```python
from build123d import *

# Parameters (mm, degrees)
F0_W     = 2
F0_H     = 15
F0_W_2   = 20
F0_H_2   = 5
F1_DEPTH = 7.5
F2_START = 2.5
F0_H_3   = 20
F0_R     = 2.5
F0_H_4   = 4.9999991059
F2_DEPTH = 5
F3_START = -2.5
F3_DEPTH = 5


with BuildPart() as f1:
    # F0 (on Front) → F1 (new body, symmetric)
    with BuildSketch(Plane.XZ):
        Polygon((10, -10), (10, 35), (-10, 35), (-10, 17), (-10, 15), (-10, -10), align=None)
        with Locations((-3, 2.5)):
            Rectangle(F0_W, F0_H, mode=Mode.SUBTRACT)
        with Locations((-3, 22.5)):
            Rectangle(F0_W, F0_H, mode=Mode.SUBTRACT)
        with Locations((3, 2.5)):
            Rectangle(F0_W, F0_H, mode=Mode.SUBTRACT)
        with Locations((3, 22.5)):
            Rectangle(F0_W, F0_H, mode=Mode.SUBTRACT)
        with Locations((0, -12.5)):
            Rectangle(F0_W_2, F0_H_2)
    extrude(amount=F1_DEPTH, both=True)

    # F0 (on Front) → F2 (join)
    with BuildSketch(Plane.XZ.offset(F2_START)):
        with Locations((0, -12.5)):
            Rectangle(F0_W_2, F0_H_2)
        with Locations((0, -25)):
            Rectangle(F0_W_2, F0_H_3)
        with Locations((-5, -25)):
            Circle(F0_R, mode=Mode.SUBTRACT)
        with Locations((5, -25)):
            Circle(F0_R, mode=Mode.SUBTRACT)
        with Locations((0, -37.499999553)):
            Rectangle(F0_W_2, F0_H_4)
    extrude(amount=F2_DEPTH)

    # F0 (on Front) → F3 (join)
    with BuildSketch(Plane.XZ.offset(F3_START)):
        with Locations((0, -12.5)):
            Rectangle(F0_W_2, F0_H_2)
        with Locations((0, -25)):
            Rectangle(F0_W_2, F0_H_3)
        with Locations((-5, -25)):
            Circle(F0_R, mode=Mode.SUBTRACT)
        with Locations((5, -25)):
            Circle(F0_R, mode=Mode.SUBTRACT)
        with Locations((0, -37.499999553)):
            Rectangle(F0_W_2, F0_H_4)
    extrude(amount=-F3_DEPTH)


solid = f1.part
```
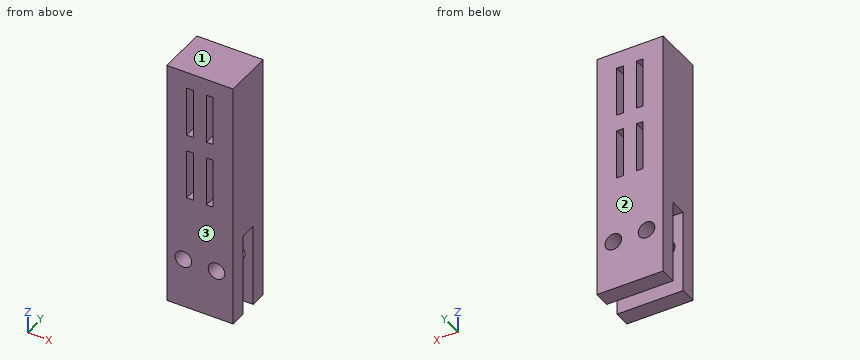
Source: CAD feature listing. Evaluate the final solid. Frame: model axes, mm. Face numbers are marked on the shaded views. Round coordinates to 2 decimals unless told otherwise and drop trailing zeros. Loops run counter-clockwise (first coordinate to the right, second up) from the corner with the lowest first, then second, coordinate; pieces in that order, holes last.
1. Section query D-D on y = -1.25. Output: boundary loops of the cut face in (x, z).
2. Section query C-C on z = -33. Output: boundary loops of the cut face in (x, y).
3. Mould query, pull axis Y, two halves, no side actions, for the marked faces 1, 2 and 3. Classes: released by +Y, released by -Y, zero draft, split by the parting line, or undercut.
4. Contact query for a flat-ended pin moving along its axis: pin 1 (2.5 mm diameter, centred on x = -2.5, y = 1, fed in from -Z). Output: stop coordinate, or through.
5. Ray query, L1, parallel to X at y = 3.75, z = 8; L2, parallel to Z at x = -2.25, y = -5.25; L3, parallel to Z at x = 2.25, y = -1.75. Return the intervals inside material, ascending.
6. Section query B-B on x = 5. Output: boundary loops of the cut face in (y, z).
7. Section query A-A on z = -25. Output: boundary loops of the cut face in (x, y), and give its area (3 significant figures).
Answers below:
1. outline: (-10, -15) - (10, -15) - (10, 35) - (-10, 35) - close; hole (-4, -5) - (-2, -5) - (-2, 10) - (-4, 10) - close; hole (-4, 15) - (-2, 15) - (-2, 30) - (-4, 30) - close; hole (2, -5) - (4, -5) - (4, 10) - (2, 10) - close; hole (2, 15) - (4, 15) - (4, 30) - (2, 30) - close
2. outline: (-10, -7.5) - (10, -7.5) - (10, -2.5) - (-10, -2.5) - close; (-10, 2.5) - (10, 2.5) - (10, 7.5) - (-10, 7.5) - close
3. face 1: zero draft
3. face 2: released by +Y
3. face 3: released by -Y
4. pin 1: stops at z = -15
5. L1: x = -10 to -4, -2 to 2, 4 to 10
5. L2: z = -40 to -5, 10 to 15, 30 to 35
5. L3: z = -15 to -5, 10 to 15, 30 to 35
6. outline: (-7.5, -40) - (-2.5, -40) - (-2.5, -27.5) - (-7.5, -27.5) - close; (-7.5, -22.5) - (-2.5, -22.5) - (-2.5, -15) - (2.5, -15) - (2.5, -22.5) - (7.5, -22.5) - (7.5, 35) - (-7.5, 35) - close; (2.5, -40) - (7.5, -40) - (7.5, -27.5) - (2.5, -27.5) - close
7. outline: (-10, -7.5) - (-7.5, -7.5) - (-7.5, -2.5) - (-10, -2.5) - close; (-10, 2.5) - (-7.5, 2.5) - (-7.5, 7.5) - (-10, 7.5) - close; (-2.5, -7.5) - (2.5, -7.5) - (2.5, -2.5) - (-2.5, -2.5) - close; (-2.5, 2.5) - (2.5, 2.5) - (2.5, 7.5) - (-2.5, 7.5) - close; (7.5, -7.5) - (10, -7.5) - (10, -2.5) - (7.5, -2.5) - close; (7.5, 2.5) - (10, 2.5) - (10, 7.5) - (7.5, 7.5) - close
7. area: 100 mm2
